Input: part model. Units: mm. Frame: model coordinates. Face numbers are marked on the shaded views. Coordinates: 2 decimals unless noted, no trailing zeros. Order: outer loops, then holes, each group sorted by start corner. A loop starts at its lowest first (then second) coordinate and runs counter-clockwise, first axis right, second up. Notation, with made-up numbers: (47, -7.75) -> (96, -7.75) arc R6 ccw to (96, 0.25) -> close; hole circle Ø10 at (17, 64). An arc over 180 degrees is marked (long way). Answer as CSV lines item,"result".
from build123d import *

# Parameters (mm, degrees)
BOX_W           = 20
BOX_H           = 20
BOX_DEPTH       = 1.5
SKETCH_R        = 2
PAD_DEPTH       = 1.5
SKETCH001_R     = 1
POCKET_DEPTH    = 5
SKETCH002_R     = 2.5
POCKET001_DEPTH = 5


with BuildPart() as part:
    # Box → Box (new body)
    with BuildSketch(Plane.XY):
        with Locations((10, 10)):
            Rectangle(BOX_W, BOX_H)
    extrude(amount=BOX_DEPTH)

    # Sketch → Pad (new body)
    with BuildSketch(Plane.XY.offset(1.5)):
        with Locations((10, 20)):
            Circle(SKETCH_R)
        with Locations((10, 0)):
            Circle(SKETCH_R)
    extrude(amount=-PAD_DEPTH)

    # Sketch001 → Pocket (cut)
    with BuildSketch(Plane.XY.offset(1.5)):
        with Locations((10, 20)):
            Circle(SKETCH001_R)
        with Locations((10, 0)):
            Circle(SKETCH001_R)
    extrude(amount=-POCKET_DEPTH, mode=Mode.SUBTRACT)

    # Sketch002 → Pocket001 (cut)
    with BuildSketch(Plane.XY.offset(1.5)):
        with Locations((0, 10)):
            Circle(SKETCH002_R)
        with Locations((20, 10)):
            Circle(SKETCH002_R)
    extrude(amount=-POCKET001_DEPTH, mode=Mode.SUBTRACT)


solid = part.part
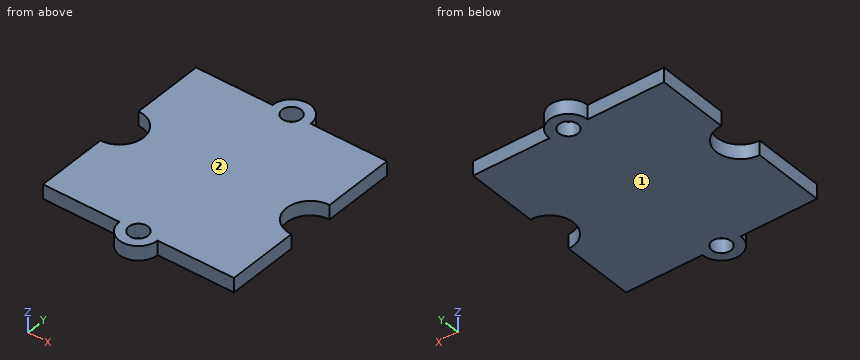
1. Cut plane B-B (z = 1.05). Return the cut outline in (x, y), plus the area to 3 significant figures.
Findings:
outline,"(0, 0) -> (8, 0) arc R2 ccw to (12, 0) -> (20, 0) -> (20, 7.5) arc R2.5 cw to (20, 12.5) -> (20, 20) -> (12, 20) arc R2 ccw to (8, 20) -> (0, 20) -> (0, 12.5) arc R2.5 cw to (0, 7.5) -> close; hole circle Ø2 at (10, 0); hole circle Ø2 at (10, 20)"
area,"387 mm2"
2. Cut plane C-C (y = 8.5). Return the cut outline in (x, z).
Findings:
outline,"(2, 0) -> (18, 0) -> (18, 1.5) -> (2, 1.5) -> close"
3. Mould query, pull axis Z, two halves, no side actions, for the marked faces 1 and 2. Classes: released by +Z, released by -Z, zero draft, split by the parting line, or undercut.
Findings:
face 1,"released by -Z"
face 2,"released by +Z"
4. Cut plane A-A (x = 10). Return the cut outline in (y, z).
Findings:
outline,"(-2, 0) -> (-1, 0) -> (-1, 1.5) -> (-2, 1.5) -> close; (1, 0) -> (19, 0) -> (19, 1.5) -> (1, 1.5) -> close; (21, 0) -> (22, 0) -> (22, 1.5) -> (21, 1.5) -> close"
5. Ray query, line 1 along Y through (x, z) = (10, 0.85); line 2 along Y through (x, z) = (19.25, 0.5); line 3 along Y through (x, z) = (13, 0.35). Return the intervals inside material, ascending.
Findings:
line 1,"y = -2 to -1, 1 to 19, 21 to 22"
line 2,"y = 0 to 7.62, 12.38 to 20"
line 3,"y = 0 to 20"
6. Contact query for a flat-ended pin moving along its axis: pin 1 (1.2 mm diameter, centred on x = 10, y = 20, fed in from -Z). Output: stop coordinate, or through.
Findings:
pin 1,"passes through"
7. Cut plane D-D (x = 15.25). Return the cut outline in (y, z), plus the area to 3 significant figures.
Findings:
outline,"(0, 0) -> (20, 0) -> (20, 1.5) -> (0, 1.5) -> close"
area,"30.0 mm2"
